```python
from build123d import *

# Parameters (mm, degrees)
F0_W          = 10
F0_H          = 30
F1_DEPTH      = 2
F3_DEPTH      = 10
F3_DEPTH_BACK = 2
F4_R          = 1.5
F4_R_2        = 19
F5_DEPTH      = 28.2830263058
F5_TAPER      = -5
F6_R          = 2.65
F7_DEPTH      = 55
F8_T1_DEPTH   = 2


# Not quite as in the source:
# - a fillet or chamfer that OpenCascade refuses, or shapes differently, is made with other operations: its cross-section is extruded or revolved along the edge and cut away or added
# - an extrude ends at something that could not be found from the text; its depth is read off the source's solid
# - a feature names something its author has since deleted; it is built from what else it names


with BuildPart() as f1:
    # F0 (on Front) → F1 (new body)
    with BuildSketch(Plane.XZ):
        with Locations((0, 4.7131987304)):
            Rectangle(F0_W, F0_H)
        with BuildLine():
            ThreePointArc((-1.5, -3.2868012696), (0, -1.7868012696), (1.5, -3.2868012696))
            Line((1.5, -3.2868012696), (1.5, -5.2868012696))
            ThreePointArc((1.5, -5.2868012696), (0, -6.7868012696), (-1.5, -5.2868012696))
            Line((-1.5, -5.2868012696), (-1.5, -3.2868012696))
        make_face(mode=Mode.SUBTRACT)
        with BuildLine():
            ThreePointArc((-1.5, 14.7131987304), (0, 16.2131987304), (1.5, 14.7131987304))
            Line((1.5, 14.7131987304), (1.5, 12.7131987304))
            ThreePointArc((1.5, 12.7131987304), (0, 11.2131987304), (-1.5, 12.7131987304))
            Line((-1.5, 12.7131987304), (-1.5, 14.7131987304))
        make_face(mode=Mode.SUBTRACT)
    extrude(amount=F1_DEPTH)

    # F2 (on face) → F3 (join, two sides)
    with BuildSketch(Plane.XZ.offset(2)) as f3_sk:
        with BuildLine():
            Line((-7.8870679483, 4.9496821465), (-5, 3.7241945098))
            Line((-5, 3.7241945098), (-5, 7.8610010163))
            ThreePointArc((-5, 7.8610010163), (-5.5824819191, 6.7769494476), (-6.807950467, 6.6643447068))
            Line((-6.807950467, 6.6643447068), (-7.1056056914, 6.7906918534))
            Line((-7.1056056914, 6.7906918534), (-7.8870679483, 4.9496821465))
        make_face()
        Polygon((5, -0.5205536523), (28.9331261898, -10.679562993), (29.7145884467, -8.8385532861), (5, 1.6521671025), align=None)
        Polygon((-5, 3.7241945098), (5, -0.5205536523), (5, 1.6521671025), (-3, 5.0479656322), (-3, 19.7131987304), (-5, 19.7131987304), (-5, 7.8610010163), align=None)
    extrude(amount=F3_DEPTH)
    extrude(f3_sk.sketch, amount=-F3_DEPTH_BACK)

    # F4 (on face) → F5 (cut, through all)
    with BuildSketch(Plane(origin=(0.5761265937, 0, 1.3572691988), x_dir=(0.9205048535, 0, -0.3907311285), z_dir=(-0.3907311285, 0, -0.9205048535))):
        with Locations((-4.1940792167, 8)):
            Circle(F4_R)
        with Locations((27.4445048224, 8)):
            Circle(F4_R)
        with Locations((11.6252128028, 24)):
            Circle(F4_R_2)
    extrude(amount=-F5_DEPTH, taper=F5_TAPER, mode=Mode.SUBTRACT)

    # F6 (on face) → F7 (cut, through all)
    with BuildSketch(Plane(origin=(1.3575888507, 0, 3.1982789057), x_dir=(0.9205048535, 0, -0.3907311285), z_dir=(0.3907311285, 0, 0.9205048535))):
        with Locations((27.4445048224, -8)):
            Circle(F6_R)
        with Locations((-4.1940792167, -8)):
            Circle(F6_R)
    extrude(amount=F7_DEPTH, mode=Mode.SUBTRACT)

    # F8: fillet of radius 28 on 2 edges, made by hand

    # F8_s2 → F8_t1 (join)
    with BuildSketch(Plane.XZ):
        with BuildLine():
            ThreePointArc((22.0555251238, -5.5874737898), (9.7786939327, 4.5355646625), (5, 19.7131987304))
            Line((5, 19.7131987304), (5, 1.6521671025))
            Line((5, 1.6521671025), (22.0555251238, -5.5874737898))
        make_face()
        with BuildLine():
            ThreePointArc((27.43600386, -10.0440722673), (16.1926256307, -7.8198466481), (5, -10.2868012696))
            Line((5, -10.2868012696), (5, -0.5205536523))
            Line((5, -0.5205536523), (27.43600386, -10.0440722673))
        make_face()
    extrude(amount=F8_T1_DEPTH)


solid = f1.part
```
Part model, mm, in its own coordinate system. A direction names the side the tool comes from. Round coordinates to 2 decimals unless told otherwise and drop trailing zeros. Loops run counter-clockwise (first coordinate to the right, second up) from the corner with the lowest first, then second, coordinate; pieces in that order, holes last. Notation, with made-up numbers: (12.5, -37) -> (59.5, -37) arc R26 cw to (59.5, -10) -> close; hole circle Ø3 at (59, 30). An arc over 180 degrees is marked (long way). Use one line per item in the form item = value. Start each with the question number.
Item 1: Band-saw the part on B-B (y = -7.25). Give the number of separate pieces and of enclosed holes in the cut face, plus the area to 3 significant figures.
Item 2: Tool access for faces 1 (the flat face through (4, -2, -5)), 2 (the flat face through (4, -2, 8)), 3 (the flat face through (-5, -6, 14)), 4 (the cylindrical face through (-0.033, -0.986, -1.787)): list every direction of +Z, -Z, +X, -X, +Y, -Y with a clear straight run to the whole face (end or side of a thin tool).
Item 3: Drill centre lines: line 1 along X through (y, z) = (-5.25, 10); line 2 along X through (y, z) = (-0.75, -6); line 3 along Y through (x, z) = (10, 3.5). Where is each one in solid material? Low to high.
Item 4: Drop flat-ended pins along their axis: pin 1 Ø2 at (y, z) = (-10.5, 10.5) entering from -X; pin 2 Ø5 at (y, z) = (-9, 16) entering from +X; pin 3 Ø4 at (y, z) = (-6.5, 2) entering from +X. Give the stop position or say it passes through.
Item 5: Band-saw the part on A-A (y = -4.25). List the corners of the cut face in (x, z), plus the area to 3 significant figures.
Item 6: Two-plate mould, pull along Z, no slides. Class faces 5 (the cylindrical face through (16.35, -0.99, -7.82)), 6 (the flat face through (-7.49, -6.08, 5.88)), 7 (the cylindrical face through (-0.033, -0.986, 16.213)): released by +Z, released by -Z, zero draft, split by the parting line, or undercut.
Data:
q1.separate_pieces = 4
q1.enclosed_holes = 0
q1.area = 56.8 mm^2
q2.face_1 = -Z, -X, -Y
q2.face_2 = +Z, +X, -Y
q2.face_3 = +Z, -X, +Y, -Y
q2.face_4 = +Y, -Y
q3.line_1 = -5 to -3
q3.line_2 = -5 to -1.32, 1.32 to 23.03
q3.line_3 = -2 to 0
q4.pin_1 = -5
q4.pin_2 = -3
q4.pin_3 = 8.01
q5.outline = (-7.89, 4.95) -> (28.93, -10.68) -> (29.71, -8.84) -> (-3, 5.05) -> (-3, 19.71) -> (-5, 19.71) -> (-5, 7.86) arc R1.3 cw to (-6.81, 6.66) -> (-7.11, 6.79) -> close
q5.area = 109 mm^2
q6.face_5 = released by -Z
q6.face_6 = released by +Z
q6.face_7 = undercut
